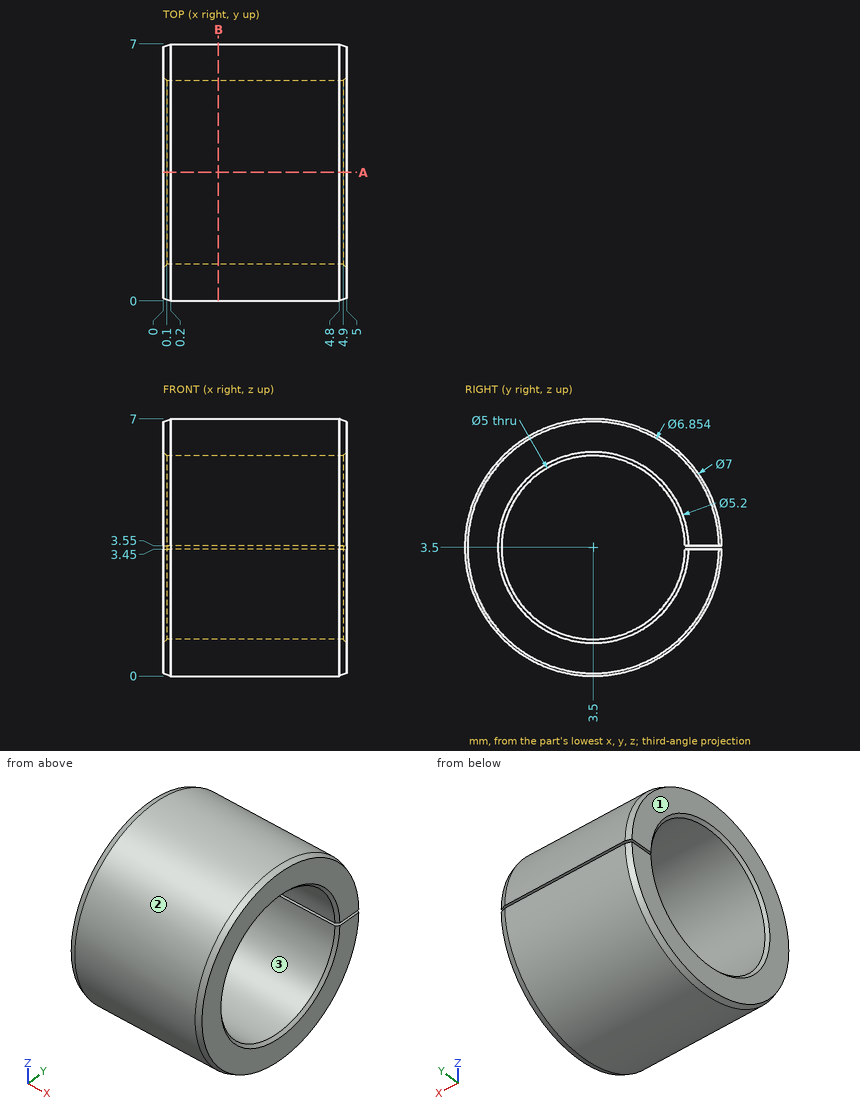
Input: dimensioned drawing with shaded views. Units: mm. Origin: part minimum x, y, z. Coordinates: 2 decimals unless noted, no trailing zeros. Write each loop counter-clockwise with the first axis right and the second up, starting at its lowest first coordinate (ties: lowest second). Pieces come first, ordered by that corner, then holes. Notation, with made-up numbers: M 78.5,60 L 117.5,60 A36 cw 117.5,99 Z; hole C 84,47 d7. An arc over 180 degrees is marked long. Answer as a JSON object with one key per item and string values. Group by question number.
(1) Section B-B on x = 1.5. Output: boundary loops of the cut face in (y, z).
(2) Section A-A on y = 3.5. Output: boundary loops of the cut face in (x, z).
(3) Ray query, line 1 along Z through (x, y) = (2.35, 3.5); line 2 along Y through (x, z) = (1.1, 3.5); line 3 along Y through (x, z) = (4.35, 5). Return the intervals inside material, ascending. Write a range as [from, to].
(4) Contact query for flat-ended pins moving along their axis: P1, Ø0.5, axis at x = 2, y = 6.5, coming from the -Z side (1 decimal); P2, Ø1.1, axis at x = 3.5, y = 6.5, coming from the +Z side; P3, Ø1.5, axis at x = 2, z = 5.5, coming from the +Y side. Output: stop coordinate, or through.
(5) Mould query, pull axis Y, two halves, no side actions, for the marked faces 1, 2 and 3. Classes: pulls with the +Y half, pulls with the -Y half, needs draft (parallel to the pull), parting line crosses it, or undercut.
Result set:
{
 "1": {"outline": "M 6,3.45 A2.5 cw long 6,3.55 L 7,3.55 A3.5 ccw long 7,3.45 Z"},
 "2": {"outline": "M 0,0.07 L 0.2,0 L 4.8,0 L 5,0.07 L 5,0.9 L 4.9,1 L 0.1,1 L 0,0.9 Z; M 0,6.1 L 0.1,6 L 4.9,6 L 5,6.1 L 5,6.93 L 4.8,7 L 0.2,7 L 0,6.93 Z"},
 "3": {"line 1": "z = [0, 1], [6, 7]", "line 2": "y = [0, 1]", "line 3": "y = [0.34, 1.5], [5.5, 6.66]"},
 "4": {"P1": "stops at z = 1.3", "P2": "stops at z = 6", "P3": "stops at y = 6.77"},
 "5": {"face 1": "needs draft", "face 2": "parting line crosses it", "face 3": "undercut"}
}
